from build123d import *

# Parameters (mm, degrees)
SKETCH1_W           = 150
SKETCH1_H           = 100
BOSS_EXTRUDE1_DEPTH = 45
CUT_EXTRUDE1_DEPTH  = 41
CUT_EXTRUDE2_DEPTH  = 101.747208398
CUT_EXTRUDE3_DEPTH  = 3
SKETCH5_R           = 2
CUT_EXTRUDE4_DEPTH  = 100.025249305
SKETCH6_W           = 150
SKETCH6_H           = 100
SKETCH6_W_2         = 130
SKETCH6_H_2         = 80
BOSS_EXTRUDE2_DEPTH = 110
SKETCH7_R           = 2
CUT_EXTRUDE5_DEPTH  = 15
SKETCH11_W          = 60
SKETCH11_H          = 100
BOSS_EXTRUDE5_DEPTH = 20
SKETCH12_R          = 2
CUT_EXTRUDE6_DEPTH  = 15
SKETCH13_R          = 2
CUT_EXTRUDE7_DEPTH  = 15
SKETCH14_R          = 2
CUT_EXTRUDE8_DEPTH  = 15
SKETCH15_W          = 50
SKETCH15_H          = 80
BOSS_EXTRUDE6_DEPTH = 110
FILLET1_R           = 3


with BuildPart() as part:
    # Sketch1 → Boss-Extrude1 (new body)
    with BuildSketch(Plane(origin=(0, 0, 0), x_dir=(1, 0, 0), z_dir=(0, 1, 0))):
        Rectangle(SKETCH1_W, SKETCH1_H)
    extrude(amount=BOSS_EXTRUDE1_DEPTH)

    # Sketch2 → Cut-Extrude1 (cut)
    with BuildSketch(Plane(origin=(0, 45, 0), x_dir=(1, 0, 0), z_dir=(0, 1, 0))):
        with BuildLine():
            Line((-6.866486348, -32.778174593), (7.778174593, -18.133513652))
            ThreePointArc((7.778174593, -18.133513652), (10.162674858, -14.564856815), (11, -10.355339059))
            Line((11, -10.355339059), (11, 10.355339059))
            ThreePointArc((11, 10.355339059), (10.162674858, 14.564856815), (7.778174593, 18.133513652))
            Line((7.778174593, 18.133513652), (-6.866486348, 32.778174593))
            ThreePointArc((-6.866486348, 32.778174593), (-10.435143185, 35.162674858), (-14.644660941, 36))
            Line((-14.644660941, 36), (-35.355339059, 36))
            ThreePointArc((-35.355339059, 36), (-39.564856815, 35.162674858), (-43.133513652, 32.778174593))
            Line((-43.133513652, 32.778174593), (-57.778174593, 18.133513652))
            ThreePointArc((-57.778174593, 18.133513652), (-60.162674858, 14.564856815), (-61, 10.355339059))
            Line((-61, 10.355339059), (-61, -10.355339059))
            ThreePointArc((-61, -10.355339059), (-60.162674858, -14.564856815), (-57.778174593, -18.133513652))
            Line((-57.778174593, -18.133513652), (-43.133513652, -32.778174593))
            ThreePointArc((-43.133513652, -32.778174593), (-39.564856815, -35.162674858), (-35.355339059, -36))
            Line((-35.355339059, -36), (-14.644660941, -36))
            ThreePointArc((-14.644660941, -36), (-10.435143185, -35.162674858), (-6.866486348, -32.778174593))
        make_face()
    extrude(amount=-CUT_EXTRUDE1_DEPTH, mode=Mode.SUBTRACT)

    # Sketch3 → Cut-Extrude2 (cut, through all)
    with BuildSketch(Plane(origin=(0, 45, 0), x_dir=(1, 0, 0), z_dir=(0, 1, 0))):
        with BuildLine():
            Line((-50.617376915, 10), (-60.617376915, 10))
            Line((-60.617376915, 10), (-60.617376915, -10))
            Line((-60.617376915, -10), (-50.617376915, -10))
            ThreePointArc((-50.617376915, -10), (-35.122065553, -25.569391642), (-13.168566779, -24.824729363))
            ThreePointArc((-13.168566779, -24.824729363), (2.5, 0), (-13.168566779, 24.824729363))
            ThreePointArc((-13.168566779, 24.824729363), (-35.122065553, 25.569391642), (-50.617376915, 10))
        make_face()
    extrude(amount=-CUT_EXTRUDE2_DEPTH, mode=Mode.SUBTRACT)

    # Sketch4 → Cut-Extrude3 (cut)
    with BuildSketch(Plane.XZ):
        Polygon((-0.366016727, 22.388617676), (-2.611382324, 24.633983273), (-5.678608771, 23.812122424), (-6.500469621, 20.744895977), (-4.255104023, 18.499530379), (-1.187877576, 19.321391229), align=None)
        Polygon((-47.388617676, 24.633983273), (-49.633983273, 22.388617676), (-48.812122424, 19.321391229), (-45.744895977, 18.499530379), (-43.499530379, 20.744895977), (-44.321391229, 23.812122424), align=None)
        Polygon((-2.611382324, -24.633983273), (-0.366016727, -22.388617676), (-1.187877576, -19.321391229), (-4.255104023, -18.499530379), (-6.500469621, -20.744895977), (-5.678608771, -23.812122424), align=None)
        Polygon((-49.633983273, -22.388617676), (-47.388617676, -24.633983273), (-44.321391229, -23.812122424), (-43.499530379, -20.744895977), (-45.744895977, -18.499530379), (-48.812122424, -19.321391229), align=None)
    extrude(amount=-CUT_EXTRUDE3_DEPTH, mode=Mode.SUBTRACT)

    # Sketch5 → Cut-Extrude4 (cut, through all)
    with BuildSketch(Plane(origin=(0, 4, 0), x_dir=(1, 0, 0), z_dir=(0, 1, 0))):
        with Locations(Location((-46.566756826, 21.566756826, 0), (0, 0, 270))):
            Circle(SKETCH5_R)
        with Locations(Location((-3.433243174, 21.566756826, 0), (0, 0, 270))):
            Circle(SKETCH5_R)
        with Locations(Location((-3.433243174, -21.566756826, 0), (0, 0, 270))):
            Circle(SKETCH5_R)
        with Locations(Location((-46.566756826, -21.566756826, 0), (0, 0, 270))):
            Circle(SKETCH5_R)
    extrude(amount=-CUT_EXTRUDE4_DEPTH, mode=Mode.SUBTRACT)

    # Sketch6 → Boss-Extrude2 (add)
    with BuildSketch(Plane.XZ):
        Rectangle(SKETCH6_W, SKETCH6_H)
        Rectangle(SKETCH6_W_2, SKETCH6_H_2, mode=Mode.SUBTRACT)
    extrude(amount=BOSS_EXTRUDE2_DEPTH)

    # Sketch7 → Cut-Extrude5 (cut)
    with BuildSketch(Plane.XZ.offset(110)):
        with Locations(Location((70, 45, 0), (0, 0, 90))):
            Circle(SKETCH7_R)
        with Locations(Location((70, -45, 0), (0, 0, 270))):
            Circle(SKETCH7_R)
        with Locations(Location((-70, -30, 0), (0, 0, 90))):
            Circle(SKETCH7_R)
        with Locations(Location((-70, 12, 0), (0, 0, 270))):
            Circle(SKETCH7_R)
    extrude(amount=-CUT_EXTRUDE5_DEPTH, mode=Mode.SUBTRACT)

    # Sketch11 → Boss-Extrude5 (add)
    with BuildSketch(Plane(origin=(-75, 0, 0), x_dir=(0, 0, -1), z_dir=(1, 0, 0))):
        with Locations((0, -32.5)):
            Rectangle(SKETCH11_W, SKETCH11_H)
    extrude(amount=-BOSS_EXTRUDE5_DEPTH)

    # Sketch12 → Cut-Extrude6 (cut)
    with BuildSketch(Plane(origin=(0, 0, -30), x_dir=(-1, 0, 0), z_dir=(0, 0, -1))):
        with Locations((85, 0)):
            Circle(SKETCH12_R)
        with Locations(Location((85, -65, 0), (0, 0, 180))):
            Circle(SKETCH12_R)
    cut_extrude6 = extrude(amount=-CUT_EXTRUDE6_DEPTH, mode=Mode.SUBTRACT)

    # Mirror1: Cut-Extrude6 across plane
    add(cut_extrude6.mirror(Plane.XY), mode=Mode.SUBTRACT)

    # Sketch13 → Cut-Extrude7 (cut)
    with BuildSketch(Plane.XZ.offset(82.5)):
        with Locations(Location((-85, 15, 0), (0, 0, 270))):
            Circle(SKETCH13_R)
        with Locations(Location((-85, -15, 0), (0, 0, 90))):
            Circle(SKETCH13_R)
    extrude(amount=-CUT_EXTRUDE7_DEPTH, mode=Mode.SUBTRACT)

    # Sketch14 → Cut-Extrude8 (cut)
    with BuildSketch(Plane(origin=(0, 45, 0), x_dir=(1, 0, 0), z_dir=(0, 1, 0))):
        with Locations(Location((60, 35, 0), (0, 0, 270))):
            Circle(SKETCH14_R)
        with Locations(Location((60, -35, 0), (0, 0, 90))):
            Circle(SKETCH14_R)
        with Locations(Location((-60, 35, 0), (0, 0, 90))):
            Circle(SKETCH14_R)
    extrude(amount=-CUT_EXTRUDE8_DEPTH, mode=Mode.SUBTRACT)

    # Sketch15 → Boss-Extrude6 (add)
    with BuildSketch(Plane.XZ):
        with Locations((40, 0)):
            Rectangle(SKETCH15_W, SKETCH15_H)
    extrude(amount=BOSS_EXTRUDE6_DEPTH)

    # Fillet1
    fillet1_edges = [part.edges().sort_by_distance(p)[0] for p in [
        (-95, -32.5, -30),
        (-85, 17.5, -30),
        (-95, -82.5, 0),
        (-85, -82.5, -30),
        (-95, -32.5, 30),
        (-85, -82.5, 30),
        (-95, 17.5, 0),
        (-85, 17.5, 30),
        (75, -32.5, 50),
        (75, -32.5, -50),
    ]]
    fillet(fillet1_edges, radius=FILLET1_R)


solid = part.part
The listing builds one solid part. Answer for the finished solid, in the listing's coordinates (mm). A direction names the side the tool comes from. Give positions to 0.01 mm unless a question says otherwise; leave off trailing zeros. Write each loop counter-clockwise with the first axis right and the second up, starting at its lowest first coordinate (ties: lowest second). Pieces come first, ordered by that corner, then holes.
Item 1: Flat-ended cylindrical pins translate along their axes: P1, Ø2.5, axis at x = -60, z = -35, coming from the +Y side; P2, Ø5, axis at x = -85, y = 0, coming from the -Z side; P3, Ø2.5, axis at x = -85, y = 0, coming from the -Z side. Find the tip coordinate at first contact, or state that the pin passes through.
Item 2: Determine the mould class of faces 5 (the flat face through (-50.35, 24.79, -25.56)), 6 (the flat face through (-75, -31, -34)), 7 (the flat face through (-83, 17.5, 0)) for opening direction X: released by +X, released by -X, zero draft, split by the parting line, or undercut.
Item 3: Section A-A, the plane y = -86.5 is taken. Write down the section's boundary in (x, z).
Item 4: Find the intervals of material crossed by line 1 along Y through (x, z) = (-85, -20); line 2 along X through (y, z) = (-100, 12); line 3 along X through (y, z) = (-77.5, -15), in increasing order.
Item 5: Section B-B, the plane y = -9.5 is taken. Write down the section's boundary in (x, z).
Item 6: Which of the six approach directions +Z, -Z, +X, -X, +Y, -Y give full straight-line access (tool end or side, diameter ignored) to faces 1 (the flat face through (-60.617, 2, 0)), 2 (the flat face through (-83, -33, -30)), 3 (the flat face through (60, 30, 35)), 4 (the cylindrical face through (-87, -75, -15))?
Completed:
1. P1: stops at y = 30
1. P2: stops at z = -30
1. P3: stops at z = -15
2. face 5: undercut
2. face 6: released by -X
2. face 7: zero draft
3. outline: (-75, -50) - (72, -50) arc R3 ccw to (75, -47) - (75, 47) arc R3 ccw to (72, 50) - (-75, 50) - close; hole (-65, -40) - (15, -40) - (15, 40) - (-65, 40) - close
4. line 1: y = -82.5 to -67, -63 to -2, 2 to 17.5
4. line 2: x = -75 to -72, -68 to -65, 15 to 75
4. line 3: x = -95 to -87, -83 to -65, 15 to 75
5. outline: (-95, -27) arc R3 ccw to (-92, -30) - (-75, -30) - (-75, -50) - (72, -50) arc R3 ccw to (75, -47) - (75, 47) arc R3 ccw to (72, 50) - (-75, 50) - (-75, 30) - (-92, 30) arc R3 ccw to (-95, 27) - close; hole (-65, -40) - (15, -40) - (15, 40) - (-65, 40) - close
6. face 1: +Y, -Y
6. face 2: -Z, -X, +Y, -Y
6. face 3: +Y
6. face 4: -Y
